CAD build for the part. Positions are in the model's coordinates, mm. A direction names the side the tool comes from. Round coordinates to 2 decimals unless told otherwise and drop trailing zeros. Loops run counter-clockwise (first coordinate to the right, second up) from the corner with the lowest first, then second, coordinate; pieces in that order, holes last. Notation, with made-up numbers: M 67.5,74 L 123.5,74 A29 ccw 123.5,95 Z; hole C 76.5,74.25 d6. An arc over 180 degrees is marked long. Use a Markdown table: item, result. Add a question column.
(1) Two-plate mould, pull along Y, no slides. Class faces 1 (the face through (217.516, -41.989, 4.056)), 2 (the face through (23, -22, -10)), 3 (the face through (18.09, -24.19, 3.52)), 4 (the face through (3, -22.6, 2.5)): released by +Y, released by -Y, zero draft, split by the parting line, or undercut.
(2) Flat gauge pins, fed straight in: P1, Ø10, axis at x = 49.5, z = -7, coming from the -Y side; P2, Ø2, axis at y = -35, z = 1.5, coming from the +X side; P3, Ø10, axis at x = 39.5, y = -33, coming from the -Z side; P4, Ø8, axis at x = 16, y = -11.5, coming from the +Z side. Where does each tip first touch, or does it go through?
(3) Wall check: L1, parallel to Y at x = 16.25, z = 2.7; L2, parallel to Z at x = 181.5, y = -6.5; L3, parallel to Z at x = 15.5, y = -43. Give the ranges that are in metal, low to high.
(4) Band-saw the part on A-A, the plane x = 157.5. Write the cut outline in (y, z).
(5) Band-saw the part on C-C, the plane x = 184. Write the cut outline in (y, z).
(6) Band-saw the part on D-D, the plane y = -9.5. Write the cut outline in (x, z), and give its area (3 significant figures).
(7) Which spindle directions (+Z, -Z, +X, -X, +Y, -Y) get a long thin tool onto all of the face, cutting with end or side? Do faces 5 (the face through (24.85, -42.71, 9.21)), 6 (the face through (23.93, -1.5, 6.48)), 7 (the face through (17, -17.4, -4.9)), 8 (the face through (16, -22, 2)), 9 (the face through (88, 0, 4)). Say none if no direction does.
(8) Band-saw the part on B-B, the plane y = -32. Write the cut outline in (x, z).
Autodesk Inventor part; units mm, degrees
ref_plane "YZ Plane" through (0, 0, 0) normal (1, 0, 0) x (0, 1, 0)
ref_plane "XZ Plane" through (0, 0, 0) normal (0, 1, 0) x (-1, 0, 0)
ref_plane "XY Plane" through (0, 0, 0) normal (0, 0, 1) x (1, 0, 0)
sketch "Sketch1" plane through (0, 0, 0) normal (0, 0, 1) x (1, 0, 0)
  line L0 (-180, 0) -> (0, 0)
  line L1 (-225, -45) -> (0, -45)
  line L2 (-180, 0) -> (-225, -45)
  line L3 (0, 0) -> (0, -45)
  dimension "d2" = 45
  dimension "d9" = 225
  dimension "d10" = 180
extrude "Extrusion1" add sketch "Sketch1" along normal blind 10
sketch "Sketch2" plane through (0, 0, 10) normal (0, 0, 1) x (1, 0, 0)
  line L0 (0, 0) -> (-180, 0)
  line L1 (-225, -45) -> (0, -45)
  line L2 (0, 0) -> (-22.5, 0)
  line L3 (-22.5, 0) -> (-22.5, -45)
  line L4 (-22.5, -45) -> (0, -45)
  line L5 (0, -45) -> (0, 0)
  dimension "d11" = 22.5
extrude "Extrusion2" cut sketch "Sketch2" against normal blind 5
sketch "Sketch3" plane through (0, 0, 5) normal (0, 0, 1) x (1, 0, 0)
  line L0 (0, -19.5) -> (0, -19.5)
  line L1 (0, -25.5) -> (0, -25.5)
  line L2 (-3, -22.5) -> (-3, -22.5)
  line L3 (0, -19.5) -> (0, -25.5)
  line L4 (0, -45) -> (-22.5, -45)
  arc A0 (0, -19.5) -> (-3, -22.5) centre (0, -22.5) ccw
  arc A1 (-3, -22.5) -> (0, -25.5) centre (0, -22.5) ccw
  point P0 (0, -22.5)
  dimension "d18" = 22.5
  dimension "d47" = 3
  dimension "d48" = 6
  dimension "d49" = 3
extrude "Extrusion3" cut sketch "Sketch3" against normal blind 5
sketch "Sketch4" plane through (0, 0, 0) normal (0, 0, -1) x (-1, 0, 0)
  circle A0 centre (22.5, -22.5) radius 7.5
  circle A1 centre (157.5, -22.5) radius 7.5
  point P0 (0, -45)
  point P1 (180, 0)
  dimension "d26" = 15
  dimension "d30" = 15
extrude "Extrusion4" add sketch "Sketch4" along normal blind 10
fillet "Fillet4" radius 5 4 edges at (-225, -45, 5) (-180, 0, 5) (-22.5, 0, 7.5) (-22.5, -45, 7.5)
chamfer "Chamfer2" distance 2 angle 45 8 edges at (-120.2145, -45, 10) (-23.9645, -43.5355, 10) (-22.5, -22.5, 10) (-23.9645, -1.4645, 10) (-102.7145, 0, 10) (-179.8423, -0.3806, 10) (-198.9645, -18.9645, 10) (-217.5483, -41.9134, 10)
sketch "Sketch5" plane through (0, 0, 5) normal (0, 0, 1) x (1, 0, 0)
  line L0 (-22.5, -40) -> (-22.5, -5)
  circle A0 centre (-16.25, -22.5) radius 2.5
  line L1 (0, -45) -> (-27.5, -45)
  point P0 (0, 0)
  dimension "d38" = 5
  dimension "d39" = 6.25
  dimension "d40" = 22.5
extrude "Extrusion5" cut sketch "Sketch5" against normal blind 3
mirror "Mirror1" about plane through (0, 0, 0) normal (1, 0, 0)
sketch "Sketch6" plane through (0, 0, 10) normal (0, 0, 1) x (1, 0, 0)
  line L0 (0, 20) -> (-240, 20)
  line L1 (-240, 20) -> (-240, -80)
  line L2 (-240, -80) -> (0, -80)
  line L3 (0, -80) -> (0, 20)
  point P0 (0, 0)
  dimension "d43" = 240
  dimension "d44" = 100
extrude "Extrusion6" cut sketch "Sketch6" against normal blind 20
properties part number "Border"
Return value:
| question | item | result |
|---|---|---|
| 1 | face 1 | split by the parting line |
| 1 | face 2 | zero draft |
| 1 | face 3 | undercut |
| 1 | face 4 | undercut |
| 2 | P1 | through |
| 2 | P2 | x = 216 |
| 2 | P3 | z = 0 |
| 2 | P4 | z = 5 |
| 3 | L1 | -45 to -25, -20 to 0 |
| 3 | L2 | 0 to 10 |
| 3 | L3 | 0 to 5 |
| 4 | outline | M -45,0 L -30,0 L -30,-10 L -15,-10 L -15,0 L 0,0 L 0,8 L -2,10 L -43,10 L -45,8 Z |
| 5 | outline | M -45,0 L -4,0 L -4,8 L -6.83,10 L -43,10 L -45,8 Z |
| 6 | outline | M 0,0 L 189.5,0 L 189.5,8 L 186.67,10 L 24.5,10 L 22.5,8 L 22.5,5 L 0,5 Z |
| 6 | area | 1,780 mm^2 |
| 7 | face 5 | +Z, -X, -Y |
| 7 | face 6 | +Z, -X, +Y |
| 7 | face 7 | -Z |
| 7 | face 8 | +Z |
| 7 | face 9 | +Z, -Z, +X, -X, +Y |
| 8 | outline | M 0,0 L 212,0 L 212,8 L 209.17,10 L 24.5,10 L 22.5,8 L 22.5,5 L 0,5 Z |
